```python
from build123d import *

# Parameters (mm, degrees)
SZKIC1_W                    = 135
SZKIC1_H                    = 65
DODANIE_WYCI_GNI_CIE1_DEPTH = 6
WYTNIJ_WYCI_GNI_CIE1_DEPTH  = 6
SZYK_LINIOWY1_COUNT         = 2
SZYK_LINIOWY1_PITCH         = 44
SZYK_LINIOWY2_COUNT         = 2
SZYK_LINIOWY2_PITCH         = 31
SZYK_LINIOWY2_COPY_1_DEPTH  = 6
SZKIC3_W                    = 15.645494432
SZKIC3_H                    = 9.425
DODANIE_WYCI_GNI_CIE2_DEPTH = 6
SZKIC4_W                    = 80.5
SZKIC4_H                    = 13
WYTNIJ_WYCI_GNI_CIE2_DEPTH  = 6


with BuildPart() as part:
    # Szkic1 → Dodanie-wyciągnięcie1 (new body)
    with BuildSketch(Plane.XY):
        with Locations((430.631728381, 262.255356576)):
            Rectangle(SZKIC1_W, SZKIC1_H)
    extrude(amount=DODANIE_WYCI_GNI_CIE1_DEPTH)

    # Szkic2 → Wytnij-wyciągnięcie1 (cut)
    with BuildSketch(Plane.XY.offset(6)):
        Polygon((363.131728381, 241.305356576), (363.131728381, 238.205356576), (371.131728381, 238.205356576), (371.131728381, 236.830356576), (373.131728381, 236.830356576), (373.131728381, 238.205356576), (374.631728381, 238.205356576), (374.631728381, 241.305356576), (373.131728381, 241.305356576), (373.131728381, 242.680356576), (371.131728381, 242.680356576), (371.131728381, 241.305356576), align=None)
    wytnij_wyci_gni_cie1 = extrude(amount=-WYTNIJ_WYCI_GNI_CIE1_DEPTH, mode=Mode.SUBTRACT)

    # Szyk liniowy1: Wytnij-wyciągnięcie1 ×2
    with Locations(*[(0, i * SZYK_LINIOWY1_PITCH, 0) for i in range(1, SZYK_LINIOWY1_COUNT)]):
        add(wytnij_wyci_gni_cie1, mode=Mode.SUBTRACT)

    # Lustro1: Wytnij-wyciągnięcie1 across plane
    add(wytnij_wyci_gni_cie1.mirror(Plane.ZY.offset(-430.631728381)), mode=Mode.SUBTRACT)

    # Szyk liniowy2: Wytnij-wyciągnięcie1 ×2
    with Locations(*[(0, i * SZYK_LINIOWY2_PITCH, 0) for i in range(1, SZYK_LINIOWY2_COUNT)]):
        add(wytnij_wyci_gni_cie1, mode=Mode.SUBTRACT)

    # Szyk liniowy2 copy 1 sketch → Szyk liniowy2 copy 1 (cut)
    with BuildSketch(Plane(origin=(861.263456762, 31, 6), x_dir=(-1, 0, 0), z_dir=(0, 0, 1))):
        Polygon((363.131728381, -241.305356576), (363.131728381, -238.205356576), (371.131728381, -238.205356576), (371.131728381, -236.830356576), (373.131728381, -236.830356576), (373.131728381, -238.205356576), (374.631728381, -238.205356576), (374.631728381, -241.305356576), (373.131728381, -241.305356576), (373.131728381, -242.680356576), (371.131728381, -242.680356576), (371.131728381, -241.305356576), align=None)
    extrude(amount=-SZYK_LINIOWY2_COPY_1_DEPTH, mode=Mode.SUBTRACT)

    # Szkic3 → Dodanie-wyciągnięcie2 (add)
    with BuildSketch(Plane.XY.offset(6)):
        with Locations((370.954475597, 272.542856576)):
            Rectangle(SZKIC3_W, SZKIC3_H)
    extrude(amount=-DODANIE_WYCI_GNI_CIE2_DEPTH)

    # Szkic4 → Wytnij-wyciągnięcie2 (cut)
    with BuildSketch(Plane.XY.offset(6)):
        with Locations((457.881728381, 288.255356576)):
            Rectangle(SZKIC4_W, SZKIC4_H)
    extrude(amount=-WYTNIJ_WYCI_GNI_CIE2_DEPTH, mode=Mode.SUBTRACT)


solid = part.part
```
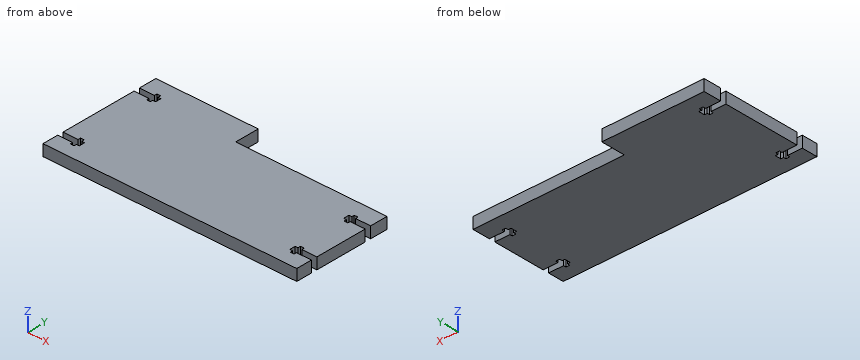
Work out the finished part from the listing and answer in its coordinate system (mm). Coordinates: 2 decimals unless noted, no trailing zeros. Write each loop counter-clockwise with the first axis right and the second up, starting at its lowest first coordinate (ties: lowest second). Pieces come first, ordered by that corner, then holes. Notation, with made-up numbers: (82.5, -1.5) - (92.5, -1.5) arc R27 cw to (92.5, 25.5) - close; hole circle Ø10 at (43, 69). An arc over 180 degrees is marked (long way). Answer as a JSON object with one key per item and string values.
Q1. Find section A-A (x = 468). Write down the section's boundary in (y, z).
Results list:
{"outline": "(229.76, 0) - (281.76, 0) - (281.76, 6) - (229.76, 6) - close"}
Q2. Given pin 1 Ø3 at (y, z) = (289.5, 3.5) entering from +X; pin 2 Ø0.9 at (y, z) = (271.5, 2) entering from +X; pin 3 Ø3 at (x, z) = (476.5, 2.5) entering from +Y, each flat-ended and moving along its own axis, determine where each tip first touches the part or whether it passes through.
Results list:
{"pin 1": "stops at x = 417.63", "pin 2": "stops at x = 486.63", "pin 3": "stops at y = 281.76"}
Q3. Consider L1, parallel to Y at x = 372, z = 4.3; L2, parallel to X at y = 242.5, z = 4.25; L3, parallel to X at y = 269, z = 2.65. Determine where each line is inside the solid, lowest interval first. Write a range as from..to.
Results list:
{"L1": "y = 229.76..236.83, 242.68..280.83, 286.68..294.76", "L2": "x = 363.13..371.13, 373.13..488.13, 490.13..498.13", "L3": "x = 363.13..488.13, 490.13..498.13"}
